from build123d import *

# Parameters (mm, degrees)
SKETCH1_R           = 1.7859375
BOSS_EXTRUDE1_DEPTH = 1.5875
FILLET1_R           = 3.571875


with BuildPart() as part:
    # Sketch1 → Boss-Extrude1 (new body)
    with BuildSketch(Plane.XY):
        with BuildLine():
            ThreePointArc((53.975, -10.998522628), (55.282397014, -6.119250683), (50.403125088, -4.811853599))
            ThreePointArc((50.403125088, -4.811853599), (52.991925359, 1.438063368), (47.625, 5.55625))
            Line((47.625, 5.55625), (40.072011619, 5.55625))
            ThreePointArc((40.072011619, 5.55625), (36.147936861, 7.178856478), (32.223862103, 5.55625))
            Line((32.223862103, 5.55625), (11.155561342, 5.55625))
            ThreePointArc((11.155561342, 5.55625), (8.470770891, 11.484009389), (5.785980441, 5.55625))
            Line((5.785980441, 5.55625), (0, 5.55625))
            ThreePointArc((0, 5.55625), (-5.55625, 0), (0, -5.55625))
            ThreePointArc((0, -5.55625), (-3.571875, -9.128125), (0, -12.7))
            ThreePointArc((0, -12.7), (8.980256121, -8.980256121), (12.7, 0))
            Line((12.7, 0), (30.833892989, 0))
            ThreePointArc((30.833892989, 0), (32.465327803, -2.537958939), (35.182607485, -3.849143997))
            Line((35.182607485, -3.849143997), (36.626477372, -6.35))
            ThreePointArc((36.626477372, -6.35), (44.337998127, -12.267257994), (53.975, -10.998522628))
        make_face()
        with BuildLine():
            ThreePointArc((0, -10.9140625), (-1.7859375, -9.128125), (0, -7.3421875))
            ThreePointArc((0, -7.3421875), (5.413228446, -4.960309977), (7.31424826, 0.639913805))
            ThreePointArc((7.31424826, 0.639913805), (8.937735019, 2.574709983), (10.872531197, 0.951223224))
            ThreePointArc((10.872531197, 0.951223224), (8.046690934, -7.37343375), (0, -10.9140625))
        make_face(mode=Mode.SUBTRACT)
        with BuildLine():
            ThreePointArc((51.29609375, -6.358520894), (53.735729745, -7.012219389), (53.08203125, -9.451855383))
            ThreePointArc((53.08203125, -9.451855383), (44.800232766, -10.542174838), (38.173144617, -5.45703125))
            ThreePointArc((38.173144617, -5.45703125), (38.826843111, -3.017395255), (41.266479106, -3.67109375))
            ThreePointArc((41.266479106, -3.67109375), (45.724702042, -7.092008528), (51.29609375, -6.358520894))
        make_face(mode=Mode.SUBTRACT)
        Circle(SKETCH1_R, mode=Mode.SUBTRACT)
        with Locations((8.470770891, 7.912134389)):
            Circle(SKETCH1_R, mode=Mode.SUBTRACT)
        with Locations((36.147936861, 1.622606478)):
            Circle(SKETCH1_R, mode=Mode.SUBTRACT)
        with Locations((47.625, 0)):
            Circle(SKETCH1_R, mode=Mode.SUBTRACT)
    extrude(amount=BOSS_EXTRUDE1_DEPTH)

    # Fillet1
    fillet1_edges = [part.edges().sort_by_distance(p)[0] for p in [
        (5.785980441, 5.55625, 0.79375),
        (11.155561342, 5.55625, 0.79375),
        (32.223862103, 5.55625, 0.79375),
        (40.072011619, 5.55625, 0.79375),
        (50.403125088, -4.811853599, 0.79375),
        (35.182607485, -3.849143997, 0.79375),
        (30.833892989, 0, 0.79375),
        (0, -5.55625, 0.79375),
    ]]
    fillet(fillet1_edges, radius=FILLET1_R)


solid = part.part
The listing builds one solid part. Answer for the finished solid, in the listing's coordinates (mm). A direction names the side the tool comes from. Give positions to 0.01 mm unless a question says otherwise; leave off trailing zeros. Answer as CSV lines item,"result".
Q1. Straight lines are drawn through the part: L1, parallel to Y at x = 47.5, z = 1.1; L2, parallel to X at y = -8, z = 0.5; L3, parallel to X at y = -8.75, z = 0.15. For each, find the intervals that lie inside material, in ascending order.
Answer key:
L1,"y = -12.7 to -10.91, -7.34 to -1.78, 1.78 to 5.56"
L2,"x = -3.39 to -1.38, 7.42 to 9.86, 37.76 to 40.2, 53.97 to 55.76"
L3,"x = -3.55 to -1.75, 6.52 to 9.2, 38.42 to 41.1, 53.76 to 55.66"
Q2. This flat-tipped pin is pushed along its axis until it touches: pin 1 Ø0.5 at (x, z) = (17.5, 0.5) entering from -Y. Where does it stop, or does it pass through?
Answer key:
pin 1,"stops at y = 0"
Q3. A cutting plane is placed at A-A, the plane z = 0.75. Count the separate pieces of the cut face and the enclosed holes in it, and give its area (3 significant figures).
Answer key:
separate pieces,"1"
enclosed holes,"6"
area,"593 mm^2"
Q4. Determine the mould class of faces 4 (the face through (45.84, 0.08, 0.78)), 5 (the face through (53.716, -6.978, 0.783)), 6 (the face through (25, 2, 1.588)), 7 (the face through (44.2, -12.23, 0.78)) for opening direction Y: pulls with the +Y half, pulls with the -Y half, needs draft (parallel to the pull), parting line crosses it, or undercut.
Answer key:
face 4,"undercut"
face 5,"undercut"
face 6,"needs draft"
face 7,"pulls with the -Y half"
Q5. Which of the six approach directions +Z, -Z, +X, -X, +Y, -Y give full straight-line access (tool end or side, diameter ignored) to faces 1 (the face through (44.916, -10.573, 0.783)), 2 (the face through (1, 5.556, 1)), 3 (the face through (36.256, -5.708, 0.783))?
Answer key:
face 1,"+Z, -Z"
face 2,"+Z, -Z, -X, +Y"
face 3,"+Z, -Z, -Y"
